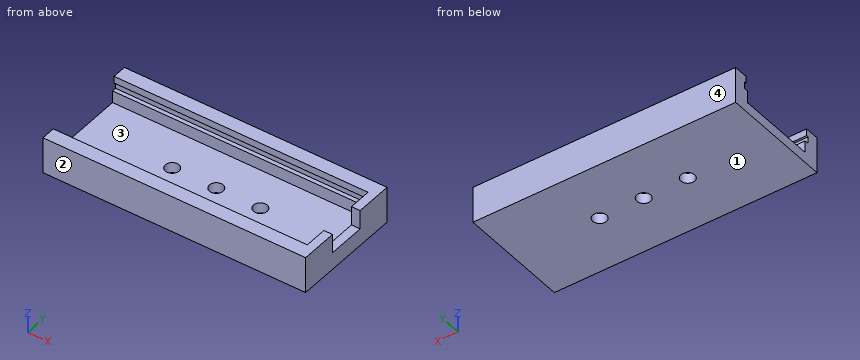
Autodesk Fusion 360 part; units mm, degrees
sketch "Main Body" plane through (0, 0, 0) normal (1, 0, 0) x (0, 1, 0)
  line L0 (0, 0) -> (16.2, 0)
  line L1 (16.2, 0) -> (16.2, 10.5)
  line L2 (16.2, 10.5) -> (12.1, 10.5)
  line L3 (12.1, 10.5) -> (12.1, 8.5)
  line L4 (12.1, 8.5) -> (12.7, 8.5)
  line L5 (12.7, 8.5) -> (12.7, 6.5)
  line L6 (12.7, 6.5) -> (11.5, 6.5)
  line L7 (11.5, 6.5) -> (11.5, 3)
  line L8 (11.5, 3) -> (0, 3)
  line L9 (0, 35) -> (0, -40) construction
  line L10 (-12.1, 10.5) -> (-12.1, 8.5)
  line L11 (-11.5, 6.5) -> (-11.5, 3)
  line L12 (-12.1, 8.5) -> (-12.7, 8.5)
  line L13 (-12.7, 6.5) -> (-11.5, 6.5)
  line L14 (-12.7, 8.5) -> (-12.7, 6.5)
  line L15 (-16.2, 10.5) -> (-12.1, 10.5)
  line L16 (-16.2, 0) -> (-16.2, 10.5)
  line L17 (0, 0) -> (-16.2, 0)
  line L18 (-11.5, 3) -> (0, 3)
  dimension "d1" = 16.2
  dimension "d4" = 4.1
  dimension "d5" = 0.6
  dimension "d6" = 2
  dimension "d9" = 4.7
  dimension "d10" = 6.5
  dimension "d11" = 2
  dimension "d16" = 3
extrude "Extrude1" add sketch "Main Body" along normal blind 76
sketch "USB Endstop" plane through (76, 0, 0) normal (1, 0, 0) x (0, 1, 0)
  line L0 (-16.2, 0) -> (16.2, 0)
  line L1 (16.2, 0) -> (16.2, 10.5)
  line L2 (16.2, 10.5) -> (12.1, 10.5)
  line L3 (12.1, 10.5) -> (12.1, 8.5)
  line L4 (12.1, 8.5) -> (12.7, 8.5)
  line L5 (12.7, 8.5) -> (12.7, 6.5)
  line L6 (12.7, 6.5) -> (11.5, 6.5)
  line L7 (11.5, 6.5) -> (11.5, 3)
  line L8 (11.5, 3) -> (-11.5, 3)
  line L9 (-11.5, 3) -> (-11.5, 6.5)
  line L10 (-11.5, 6.5) -> (-12.7, 6.5)
  line L11 (-12.7, 6.5) -> (-12.7, 8.5)
  line L12 (-12.7, 8.5) -> (-12.1, 8.5)
  line L13 (-12.1, 8.5) -> (-12.1, 10.5)
  line L14 (-12.1, 10.5) -> (-16.2, 10.5)
  line L15 (-16.2, 10.5) -> (-16.2, 0)
  line L16 (0, 5) -> (5.5, 5)
  line L17 (5.5, 5) -> (5.5, 10.5)
  line L18 (5.5, 10.5) -> (12.1, 10.5)
  line L19 (0, 12) -> (0, -4) construction
  line L20 (-5.5, 5) -> (-5.5, 10.5)
  line L21 (-5.5, 10.5) -> (-12.1, 10.5)
  line L22 (0, 5) -> (-5.5, 5)
  dimension "d14" = 5.5
  dimension "d15" = 5
extrude "Extrude2" add sketch "USB Endstop" against normal blind 2.5 contours L3 L4 L5 L6 L7 L8 L9 L10 L11 L12 L13 L16 L17 L18 L20 L21 L22
sketch "DIN Holes" plane through (0, 0, 0) normal (0, 0, -1) x (1, 0, 0)
  line L0 (0, 16.2) -> (0, -16.2)
  line L1 (0, -16.2) -> (76, -16.2)
  line L2 (76, -16.2) -> (76, 16.2)
  line L3 (76, 16.2) -> (0, 16.2)
  line L4 (0, 16) -> (76, -16.2) construction
  line L5 (76.7439, 16.2) -> (0, -16.2) construction
  circle A0 centre (38.372, 0) radius 2
  circle A1 centre (25.622, 0) radius 2
  circle A2 centre (51.122, 0) radius 2
  dimension "d20" = 4
  dimension "d23" = 12.75
  dimension "d24" = 0
extrude "Extrude3" cut sketch "DIN Holes" against normal up to surface (3 mm away) contours A0 | A1 | A2
The model under review builds one solid part; all positions refer to its coordinate system, in mm. Face numbers are marked on the shaded views. Coordinates: 2 decimals unless noted, no trailing zeros. Order: outer loops, then holes, each group sorted by start corner. A loop starts at its lowest first (then second) coordinate and runs counter-clockwise, first axis right, second up. Notation, with made-up numbers: M 22.5,9.25 L 70.5,9.25 A24 ccw 70.5,22.25 Z; hole C 87,61.5 d10. An arc over 180 degrees is marked long. One line per question, with ' | ' between items.
(1) Add section C-C, the plane x = 70. Write out the cut boundary in (y, z), then the cut area to 4 significant figures.
Geometry results:
outline: M -16.2,0 L 16.2,0 L 16.2,10.5 L 12.1,10.5 L 12.1,8.5 L 12.7,8.5 L 12.7,6.5 L 11.5,6.5 L 11.5,3 L -11.5,3 L -11.5,6.5 L -12.7,6.5 L -12.7,8.5 L -12.1,8.5 L -12.1,10.5 L -16.2,10.5 Z | area: 160.5 mm²
(2) Add section A-A, the plane z = 2.25. Write out the cut boundary in (x, y).
Geometry results:
outline: M 0,-16.2 L 76,-16.2 L 76,16.2 L 0,16.2 Z; hole C 25.62,0 d4; hole C 38.37,0 d4; hole C 51.12,0 d4
(3) For probe 1 along X at (y, z) = (0, 0.95); probe 2 along Y at (x, z) = (28.5, 9.5); probe 3 along Y at (x, z) = (35.5, 5.5), list the stretches that pass through material, from the lowest coordinate up. Write a range as from..to.
Geometry results:
probe 1: x = 0..23.62, 27.62..36.37, 40.37..49.12, 53.12..76 | probe 2: y = -16.2..-12.1, 12.1..16.2 | probe 3: y = -16.2..-11.5, 11.5..16.2
(4) The part is to be moulded in two halves that separate along Y. For the marked faces 1, 2, 3 and 4, say which applies: +Y half, -Y half, draft (parallel to the pull), parting line (faces both ways), or undercut.
Geometry results:
face 1: draft | face 2: -Y half | face 3: undercut | face 4: +Y half
(5) Insertion check: pin 1 (8 mm diameter, centred on x = 66, y = -2, fed in from -Z); pin 2 (4.5 mm diameter, centred on x = 51.122, y = 0, fed in from +Z). Each pin has a flat end and moves straight along its axis. Give the tip position at first contact, or say it passes through.
Geometry results:
pin 1: stops at z = 0 | pin 2: stops at z = 3
(6) Add section B-B, the plane y = 0. Write out the cut boundary in (x, z).
Geometry results:
outline: M 0,0 L 23.62,0 L 23.62,3 L 0,3 Z; M 27.62,0 L 36.37,0 L 36.37,3 L 27.62,3 Z; M 40.37,0 L 49.12,0 L 49.12,3 L 40.37,3 Z; M 53.12,0 L 76,0 L 76,5 L 73.5,5 L 73.5,3 L 53.12,3 Z
(7) Add section D-D, the plane x = 38. Write out the cut boundary in (y, z).
Geometry results:
outline: M -16.2,0 L -1.97,0 L -1.97,3 L -11.5,3 L -11.5,6.5 L -12.7,6.5 L -12.7,8.5 L -12.1,8.5 L -12.1,10.5 L -16.2,10.5 Z; M 1.97,0 L 16.2,0 L 16.2,10.5 L 12.1,10.5 L 12.1,8.5 L 12.7,8.5 L 12.7,6.5 L 11.5,6.5 L 11.5,3 L 1.97,3 Z
